Geometry check sheet. Reference: the model listing, model coordinates, mm. Face numbers are marked on the shaded views. Round coordinates to 2 decimals unless told otherwise and drop trailing zeros. Loops run counter-clockwise (first coordinate to the right, second up) from the corner with the lowest first, then second, coordinate; pieces in that order, holes last. Notation, with made-up numbers: M 2.25,72.25 L 7.25,72.25 A30 ccw 7.25,110.25 Z; hole C 34,41 d1. An arc over 180 degrees is marked long. Answer in a Markdown table with one row per item. Add a question column.
```python
from build123d import *

# Parameters (mm, degrees)
SKETCH_1_W          = 50
SKETCH_1_H          = 30
EXTRUDE_1_DEPTH     = 2.4
SKETCH_2_R          = 1.65
CUT_EXTRUDE_1_DEPTH = 59.35888964
CHAMFER_1_SIZE      = 2
FILLET_1_R          = 2
CHAMFER_2_SIZE      = 1
CHAMFER_3_SIZE      = 0.4


with BuildPart() as part:
    # 草图1 → 凸台-拉伸1 (new body)
    with BuildSketch(Plane(origin=(0, 0, 0), x_dir=(1, 0, 0), z_dir=(0, 1, 0))):
        with Locations((25, 15)):
            Rectangle(SKETCH_1_W, SKETCH_1_H)
    extrude(amount=EXTRUDE_1_DEPTH)

    # 草图2 → 切除-拉伸1 (cut, through all)
    with BuildSketch(Plane(origin=(0, 2.4, 0), x_dir=(1, 0, 0), z_dir=(0, 1, 0))):
        with Locations(Location((13, 6, 0), (0, 0, 270))):
            Circle(SKETCH_2_R)
        with Locations(Location((37, 6, 0), (0, 0, 270))):
            Circle(SKETCH_2_R)
        with Locations(Location((13, 22, 0), (0, 0, 270))):
            Circle(SKETCH_2_R)
        with Locations(Location((37, 22, 0), (0, 0, 270))):
            Circle(SKETCH_2_R)
    extrude(amount=-CUT_EXTRUDE_1_DEPTH, mode=Mode.SUBTRACT)

    # 倒角1
    chamfer_1_edges = [part.edges().sort_by_distance(p)[0] for p in [
        (13, 2.4, -7.65),
        (37, 2.4, -23.65),
        (37, 2.4, -7.65),
        (13, 2.4, -23.65),
    ]]
    chamfer(chamfer_1_edges, length=CHAMFER_1_SIZE)

    # 圆角1
    fillet_1_edges = [part.edges().sort_by_distance(p)[0] for p in [
        (0, 1.2, -30),
        (50, 1.2, -30),
        (50, 1.2, 0),
        (0, 1.2, 0),
    ]]
    fillet(fillet_1_edges, radius=FILLET_1_R)

    # 倒角2
    chamfer_2_edges = [part.edges().sort_by_distance(p)[0] for p in [
        (25, 2.4, -30),
        (50, 2.4, -15),
        (0, 2.4, -15),
        (25, 2.4, 0),
        (0.585786438, 2.4, -29.414213562),
        (0.585786438, 2.4, -0.585786438),
        (49.414213562, 2.4, -0.585786438),
        (49.414213562, 2.4, -29.414213562),
    ]]
    chamfer(chamfer_2_edges, length=CHAMFER_2_SIZE)

    # 倒角3
    chamfer_3_edges = [part.edges().sort_by_distance(p)[0] for p in [
        (25, 0, -30),
        (0, 0, -15),
        (50, 0, -15),
        (25, 0, 0),
        (0.585786438, 0, -29.414213562),
        (0.585786438, 0, -0.585786438),
        (49.414213562, 0, -0.585786438),
        (49.414213562, 0, -29.414213562),
    ]]
    chamfer(chamfer_3_edges, length=CHAMFER_3_SIZE)


solid = part.part
```
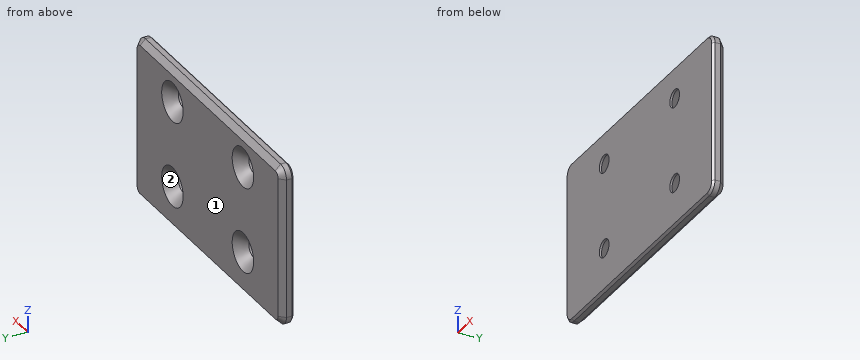
1) Go/stop test with flat-tipped pins: pin 1 (1.5 mm diameter, centred on x = 13.5, z = -4, fed in from +Y); pin 2 (3 mm diameter, centred on x = 37, z = -6, fed in from +Y). Record where each tip stops, or that it passes through.
2) Cross-section at A-A, the plane z = -22. Record the boundary of the cut face in (x, y), plus the area to 3 significant figures.
3) Draft check along Z on the marked faces 1 and 2. Enter one of: +Z half, -Z half, draft (parallel to the pull), parting line (faces both ways), or undercut.
4) Thickness scan on L1, parallel to X at y = 2.05, z = -8.75; L2, parallel to Z at x = 34, y = 2.2; L3, parallel to Y at x = 37, z = -8.25. Record the ranges inside material, lowest first. Write a range as [from, to].
5) Cross-section at B-B, the plane x = 13. Record the boundary of the cut face in (y, z).
Worked answers:
| question | item | result |
|---|---|---|
| 1 | pin 1 | stops at y = 1.56 |
| 1 | pin 2 | passes through |
| 2 | outline | M 0,0.4 L 0.4,0 L 11.35,0 L 11.35,0.4 L 9.35,2.4 L 1,2.4 L 0,1.4 Z; M 14.65,0 L 35.35,0 L 35.35,0.4 L 33.35,2.4 L 16.65,2.4 L 14.65,0.4 Z; M 38.65,0 L 49.6,0 L 50,0.4 L 50,1.4 L 49,2.4 L 40.65,2.4 L 38.65,0.4 Z |
| 2 | area | 95.0 mm2 |
| 3 | face 1 | draft |
| 3 | face 2 | undercut |
| 4 | L1 | x = [0.65, 11.18], [14.82, 35.18], [38.82, 49.35] |
| 4 | L2 | z = [-29.2, -23.7], [-20.3, -7.7], [-4.3, -0.8] |
| 4 | L3 | y = [0, 1] |
| 5 | outline | M 0,-29.6 L 0.4,-30 L 1.4,-30 L 2.4,-29 L 2.4,-25.65 L 0.4,-23.65 L 0,-23.65 Z; M 0,-20.35 L 0.4,-20.35 L 2.4,-18.35 L 2.4,-9.65 L 0.4,-7.65 L 0,-7.65 Z; M 0,-4.35 L 0.4,-4.35 L 2.4,-2.35 L 2.4,-1 L 1.4,0 L 0.4,0 L 0,-0.4 Z |
